Build history of the part. All positions in model axes, mm. A direction names the side the tool comes from. Coordinates: 2 decimals unless noted, no trailing zeros. Write each loop counter-clockwise with the first axis right and the second up, starting at its lowest first coordinate (ties: lowest second). Pieces come first, ordered by that corner, then holes.
```python
from build123d import *

# Parameters (mm, degrees)
SKETCH1_R           = 6.5
BOSS_EXTRUDE1_DEPTH = 110
SKETCH6_R           = 2.5
BOSS_EXTRUDE2_DEPTH = 2.5
SKETCH7_R           = 2.65
CUT_EXTRUDE1_DEPTH  = 3
SKETCH9_OUTSIDE_W   = 37.798
SKETCH9_OUTSIDE_H   = 37.798
SKETCH9_OUTSIDE_R   = 5.45
CUT_EXTRUDE2_DEPTH  = 107.5
SKETCH10_R          = 5.75
BOSS_EXTRUDE3_DEPTH = 10
JOIN1_START         = 90
JOIN1_OUTLINE_R     = 5.75
JOIN1_OUTLINE_R_2   = 1.5
JOIN1_DEPTH         = 20


# Read off the part's stored shape, not the designer's step: Join1
with BuildPart() as part:
    # Sketch1 → Boss-Extrude1 (new body)
    with BuildSketch(Plane.XY):
        Circle(SKETCH1_R)
    extrude(amount=BOSS_EXTRUDE1_DEPTH)

    # Sketch6 → Boss-Extrude2 (add)
    with BuildSketch(Plane(origin=(0, 0, 0), x_dir=(-1, 0, 0), z_dir=(0, 0, -1))):
        Circle(SKETCH6_R)
    extrude(amount=BOSS_EXTRUDE2_DEPTH)

    # Sketch7 → Cut-Extrude1 (cut)
    with BuildSketch(Plane.XY.offset(110)):
        Circle(SKETCH7_R)
    extrude(amount=-CUT_EXTRUDE1_DEPTH, mode=Mode.SUBTRACT)

    # Sketch9 outside → Cut-Extrude2 (cut)
    with BuildSketch(Plane.XY.offset(110)):
        Rectangle(SKETCH9_OUTSIDE_W, SKETCH9_OUTSIDE_H)
        Circle(SKETCH9_OUTSIDE_R, mode=Mode.SUBTRACT)
    extrude(amount=-CUT_EXTRUDE2_DEPTH, mode=Mode.SUBTRACT)

    # Sketch10 → Boss-Extrude3 (add)
    with BuildSketch(Plane.XY.offset(110)):
        Circle(SKETCH10_R)
    extrude(amount=-BOSS_EXTRUDE3_DEPTH)

    # Join1 outline → Join1 (add)
    with BuildSketch(Plane.XY.offset(JOIN1_START)):
        with BuildLine():
            Line((-9.619925066, 6.956270405), (-9.592077276, 5.322159982))
            Line((-9.592077276, 5.322159982), (-8.170365761, 4.533323955))
            ThreePointArc((-8.170365761, 4.533323955), (-4.533323955, -8.170365761), (8.170365761, -4.533323955))
            Line((8.170365761, -4.533323955), (8.6389607, -3.688779845))
            ThreePointArc((8.6389607, -3.688779845), (9.371491926, 0.643333346), (8.053841212, 4.834705829))
            Line((8.053841212, 4.834705829), (9.405164385, 5.645902605))
            Line((9.405164385, 5.645902605), (9.377316595, 7.280013028))
            ThreePointArc((9.377316595, 7.280013028), (18.552203658, 16.773030292), (9.059186394, 25.947917355))
            Line((9.059186394, 25.947917355), (8.661829886, 25.941145781))
            ThreePointArc((8.661829886, 25.941145781), (4.239851168, 24.521014764), (1.047885733, 21.147289146))
            Line((1.047885733, 21.147289146), (-0.373825781, 21.936125173))
            Line((-0.373825781, 21.936125173), (-1.725148954, 21.124928398))
            ThreePointArc((-1.725148954, 21.124928398), (-4.771249912, 24.237629458), (-8.893805616, 25.641970375))
            Line((-8.893805616, 25.641970375), (-9.938055267, 25.624174732))
            ThreePointArc((-9.938055267, 25.624174732), (-19.11294233, 16.131157468), (-9.619925066, 6.956270405))
        make_face()
        Circle(JOIN1_OUTLINE_R, mode=Mode.SUBTRACT)
        with Locations((-9.778990166, 16.290222568)):
            Circle(JOIN1_OUTLINE_R, mode=Mode.SUBTRACT)
        with Locations((-0.187584514, 11.00747351)):
            Circle(JOIN1_OUTLINE_R_2, mode=Mode.SUBTRACT)
        with Locations((9.218251494, 16.613965192)):
            Circle(JOIN1_OUTLINE_R, mode=Mode.SUBTRACT)
    extrude(amount=JOIN1_DEPTH)


solid = part.part
```
1. 3-axis set-ups, long thin cutter, end or side, ignore diameter. For faces 1 (the face through (3, 0, 0)), 2 (the face through (-4.719, 24.205, 99.86)), 3 (the face through (-0.75, 5.7, 94.93)): which of +Z, -Z, +X, -X, +Y, -Y reach the whole face in a straight line?
Computed values:
face 1: -Z
face 2: +Z, -Z, +Y
face 3: none
2. Saw through at B-B on y = 0. List the corners of the cut face in (x, z), plus the area to 3 significant figures.
Computed values:
outline: (-9.34, 90) - (-5.75, 90) - (-5.75, 100) - (-5.45, 100) - (-5.45, 2.5) - (-6.5, 2.5) - (-6.5, 0) - (-2.5, 0) - (-2.5, -2.5) - (2.5, -2.5) - (2.5, 0) - (6.5, 0) - (6.5, 2.5) - (5.45, 2.5) - (5.45, 100) - (5.75, 100) - (5.75, 90) - (9.39, 90) - (9.39, 110) - (-9.34, 110) - close
area: 1,370 mm2
3. Flat gauge pins, fed straight in: pin 1 (12 mm diameter, centred on y = 6.5, z = 78.5, fed in from -X); pin 2 (7 mm diameter, centred on x = -9.78, y = 16.29, fed in from +Z); pin 3 (1 mm diameter, centred on x = -0.5, z = 71, fed in from -Y); pin 4 (8 mm diameter, centred on y = -3.5, z = 33, fed in from +X). Where does each tip first touch, or does it go through?
Computed values:
pin 1: stops at x = -5.43
pin 2: passes through
pin 3: stops at y = -5.45
pin 4: stops at x = 5.45
4. Probe line 1 along X through (y, z) = (-3.5, 98.5); line 2 along Y through (x, z) = (0, 95.25); line 3 along Z through (x, y) = (8.5, 24.5). List the from-to ranges inside material, lowest first.
Computed values:
line 1: x = -8.66 to -4.56, -4.18 to 4.18, 4.56 to 8.72
line 2: y = -9.34 to -5.75, -5.45 to 5.45, 5.75 to 9.52, 12.5 to 21.73
line 3: z = 90 to 110
5. Saw through at A-A on x = -13. List the corners of the cut face in (y, z), plus the area to 3 significant figures.
Computed values:
outline: (7.53, 90) - (11.53, 90) - (11.53, 110) - (7.53, 110) - close; (21.05, 90) - (25.05, 90) - (25.05, 110) - (21.05, 110) - close
area: 160 mm2
6. Saw through at C-C on z = 28. List the corners of the cut face in (x, y).
Computed values:
outline: circle Ø10.9 at (0, 0)
7. Mould opens along Y. For faces 4 (the face through (-1, 9, 90)), 5 (the face through (-4.71, -8.07, 99.86)), 6 (the face through (0.54, -2.44, -1.23)) say: +Y half, -Y half, draft (parallel to the pull), parting line (faces both ways), or undercut.
Computed values:
face 4: draft
face 5: undercut
face 6: parting line
